Verification items for the finished model (mm, model axes). Give positions to 0.01 mm unless a question says otherwise; leave off trailing zeros. Loops run counter-clockwise (first coordinate to the right, second up) from the corner with the lowest first, then second, coordinate; pieces in that order, holes last. Notation, with made-up numbers: (40, 58.25) - (57, 58.25) arc R13 ccw to (57, 71.25) - close; hole circle Ø5 at (18.25, 74). An arc over 180 degrees is marked (long way). Answer in a Markdown table with one row per item.
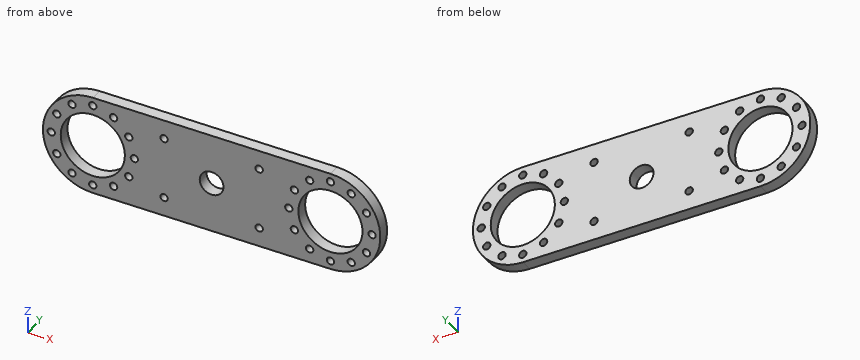
```python
from build123d import *

# Parameters (mm, degrees)
SKETCH_1_R          = 13.5
SKETCH_1_R_2        = 1.55
EXTRUDE_1_DEPTH     = 5
SKETCH_2_R          = 5
CUT_EXTRUDE_1_DEPTH = 5


with BuildPart() as part:
    # 草图1 → 凸台-拉伸1 (new body)
    with BuildSketch(Plane(origin=(0, 0, 0), x_dir=(1, 0, 0), z_dir=(0, 1, 0))):
        with BuildLine():
            Line((-50, 21), (50, 21))
            ThreePointArc((50, 21), (71, 0), (50, -21))
            Line((50, -21), (-50, -21))
            ThreePointArc((-50, -21), (-71, 0), (-50, 21))
        make_face()
        with Locations(Location((-50, 0, 0), (0, 0, 270))):
            Circle(SKETCH_1_R, mode=Mode.SUBTRACT)
        with Locations(Location((-50, 17.5, 0), (0, 0, 270))):
            Circle(SKETCH_1_R_2, mode=Mode.SUBTRACT)
        with Locations(Location((-20, 13, 0), (0, 0, 270))):
            Circle(SKETCH_1_R_2, mode=Mode.SUBTRACT)
        with Locations(Location((-20, -13, 0), (0, 0, 270))):
            Circle(SKETCH_1_R_2, mode=Mode.SUBTRACT)
        with Locations(Location((-41.25, 15.155444566, 0), (0, 0, 270))):
            Circle(SKETCH_1_R_2, mode=Mode.SUBTRACT)
        with Locations(Location((-34.844555434, 8.75, 0), (0, 0, 270))):
            Circle(SKETCH_1_R_2, mode=Mode.SUBTRACT)
        with Locations(Location((-32.5, 0, 0), (0, 0, 270))):
            Circle(SKETCH_1_R_2, mode=Mode.SUBTRACT)
        with Locations(Location((-34.844555434, -8.75, 0), (0, 0, 270))):
            Circle(SKETCH_1_R_2, mode=Mode.SUBTRACT)
        with Locations(Location((-41.25, -15.155444566, 0), (0, 0, 270))):
            Circle(SKETCH_1_R_2, mode=Mode.SUBTRACT)
        with Locations(Location((-50, -17.5, 0), (0, 0, 270))):
            Circle(SKETCH_1_R_2, mode=Mode.SUBTRACT)
        with Locations(Location((-58.75, -15.155444566, 0), (0, 0, 270))):
            Circle(SKETCH_1_R_2, mode=Mode.SUBTRACT)
        with Locations(Location((-65.155444566, -8.75, 0), (0, 0, 270))):
            Circle(SKETCH_1_R_2, mode=Mode.SUBTRACT)
        with Locations(Location((-67.5, 0, 0), (0, 0, 270))):
            Circle(SKETCH_1_R_2, mode=Mode.SUBTRACT)
        with Locations(Location((-65.155444566, 8.75, 0), (0, 0, 270))):
            Circle(SKETCH_1_R_2, mode=Mode.SUBTRACT)
        with Locations(Location((-58.75, 15.155444566, 0), (0, 0, 270))):
            Circle(SKETCH_1_R_2, mode=Mode.SUBTRACT)
        with Locations(Location((58.75, 15.155444566, 0), (0, 0, 90))):
            Circle(SKETCH_1_R_2, mode=Mode.SUBTRACT)
        with Locations(Location((65.155444566, 8.75, 0), (0, 0, 90))):
            Circle(SKETCH_1_R_2, mode=Mode.SUBTRACT)
        with Locations(Location((67.5, 0, 0), (0, 0, 90))):
            Circle(SKETCH_1_R_2, mode=Mode.SUBTRACT)
        with Locations(Location((65.155444566, -8.75, 0), (0, 0, 90))):
            Circle(SKETCH_1_R_2, mode=Mode.SUBTRACT)
        with Locations(Location((58.75, -15.155444566, 0), (0, 0, 90))):
            Circle(SKETCH_1_R_2, mode=Mode.SUBTRACT)
        with Locations(Location((50, -17.5, 0), (0, 0, 90))):
            Circle(SKETCH_1_R_2, mode=Mode.SUBTRACT)
        with Locations(Location((41.25, -15.155444566, 0), (0, 0, 90))):
            Circle(SKETCH_1_R_2, mode=Mode.SUBTRACT)
        with Locations(Location((34.844555434, -8.75, 0), (0, 0, 90))):
            Circle(SKETCH_1_R_2, mode=Mode.SUBTRACT)
        with Locations(Location((32.5, 0, 0), (0, 0, 90))):
            Circle(SKETCH_1_R_2, mode=Mode.SUBTRACT)
        with Locations(Location((41.25, 15.155444566, 0), (0, 0, 90))):
            Circle(SKETCH_1_R_2, mode=Mode.SUBTRACT)
        with Locations(Location((20, -13, 0), (0, 0, 90))):
            Circle(SKETCH_1_R_2, mode=Mode.SUBTRACT)
        with Locations(Location((20, 13, 0), (0, 0, 90))):
            Circle(SKETCH_1_R_2, mode=Mode.SUBTRACT)
        with Locations(Location((50, 17.5, 0), (0, 0, 90))):
            Circle(SKETCH_1_R_2, mode=Mode.SUBTRACT)
        with Locations(Location((50, 0, 0), (0, 0, 90))):
            Circle(SKETCH_1_R, mode=Mode.SUBTRACT)
        with Locations(Location((34.844555434, 8.75, 0), (0, 0, 90))):
            Circle(SKETCH_1_R_2, mode=Mode.SUBTRACT)
    extrude(amount=EXTRUDE_1_DEPTH)

    # 草图2 → 切除-拉伸1 (cut)
    with BuildSketch(Plane(origin=(0, 5, 0), x_dir=(1, 0, 0), z_dir=(0, 1, 0))):
        with Locations(Location((0, 0, 0), (0, 0, 270))):
            Circle(SKETCH_2_R)
    extrude(amount=-CUT_EXTRUDE_1_DEPTH, mode=Mode.SUBTRACT)


solid = part.part
```
Q1. Thickness scan on line 1 (X direction, y = 0.55, z = -18.5); line 2 (Z direction, x = 64, y = 1.6); line 3 (Z direction, x = 49, y = 0.3). Record the ranges inside material, lowest first.
Completed:
| item | result |
|---|---|
| line 1 | -59.94 to -51.18, -48.82 to 48.82, 51.18 to 59.94 |
| line 2 | -15.65 to -9.78, -7.72 to 7.72, 9.78 to 15.65 |
| line 3 | -21 to -18.68, -16.32 to -13.46, 13.46 to 16.32, 18.68 to 21 |
Q2. Sectioned sample at A-A (z = 0). Give the number of separate pieces and of enclosed holes in the cut face, and give its area (3 significant figures).
Completed:
| item | result |
|---|---|
| separate pieces | 8 |
| enclosed holes | 0 |
| area | 328 mm^2 |
Q3. Sectioned sample at C-C (x = -20). Record the cut outline in (y, z).
Completed:
| item | result |
|---|---|
| outline | (0, -21) - (5, -21) - (5, -14.55) - (0, -14.55) - close; (0, -11.45) - (5, -11.45) - (5, 11.45) - (0, 11.45) - close; (0, 14.55) - (5, 14.55) - (5, 21) - (0, 21) - close |
Q4. Go/stop test with flat-tipped pins: P1, Ø3, axis at x = 34.84, z = -8.75, coming from the -Y side; P2, Ø3.5, axis at x = 20, z = -13, coming from the -Y side; P3, Ø1, axis at y = 3.5, z = -12, coming from the -X side. Record where each tip stops, or that it passes through.
Completed:
| item | result |
|---|---|
| P1 | through |
| P2 | y = 0 |
| P3 | x = -67.57 |
Q5. Sectioned sample at B-B (x = 41.25). Record the cut outline in (y, z), and give its area (3 significant figures).
Completed:
| item | result |
|---|---|
| outline | (0, -21) - (5, -21) - (5, -16.71) - (0, -16.71) - close; (0, -13.61) - (5, -13.61) - (5, -10.28) - (0, -10.28) - close; (0, 10.28) - (5, 10.28) - (5, 13.61) - (0, 13.61) - close; (0, 16.71) - (5, 16.71) - (5, 21) - (0, 21) - close |
| area | 76.2 mm^2 |
